from build123d import *

# Parameters (mm, degrees)
SKETCH_R        = 70
SKETCH_R_2      = 57.25
PAD_DEPTH       = 15
SKETCH001_R     = 4
SKETCH002_W     = 40
SKETCH002_H     = 40
PAD001_DEPTH    = 5
SKETCH003_R     = 2.5
POCKET_DEPTH    = 5
FILLET_R        = 18
FILLET001_R     = 11
SKETCH004_R     = 58
POCKET001_DEPTH = 15.001
SKETCH005_R     = 71
POCKET002_DEPTH = 7
SKETCH006_R     = 4
SKETCH007_R     = 105
SKETCH007_R_2   = 70
POCKET003_DEPTH = 5


with BuildPart() as part:
    # Sketch → Pad (new body)
    with BuildSketch(Plane.XY):
        Circle(SKETCH_R)
        Circle(SKETCH_R_2, mode=Mode.SUBTRACT)
    extrude(amount=PAD_DEPTH)

    # Sketch001 → Groove (revolve, cut)
    with BuildSketch(Plane.XZ):
        with Locations((63.625, 16)):
            Circle(SKETCH001_R)
    revolve(axis=Axis((0, 0, 0), (0, 0, 1)), mode=Mode.SUBTRACT)

    # Sketch002 (on Face2 of Groove) → Pad001 (join)
    with BuildSketch(Plane(origin=(0, 0, 0), x_dir=(1, 0, 0), z_dir=(0, 0, -1))):
        with Locations((82, 0)):
            Rectangle(SKETCH002_W, SKETCH002_H)
        with Locations((-82, 0)):
            Rectangle(SKETCH002_W, SKETCH002_H)
        with Locations((0, 82)):
            Rectangle(SKETCH002_W, SKETCH002_H)
        with Locations((0, -82)):
            Rectangle(SKETCH002_W, SKETCH002_H)
    extrude(amount=-PAD001_DEPTH)

    # Sketch003 (on Face13 of Pad001) → Pocket (cut)
    with BuildSketch(Plane.XY.offset(5)):
        with Locations((-86.25, 0)):
            Circle(SKETCH003_R)
        with Locations((0, -86.25)):
            Circle(SKETCH003_R)
        with Locations((86.25, 0)):
            Circle(SKETCH003_R)
        with Locations((0, 86.25)):
            Circle(SKETCH003_R)
    extrude(amount=-POCKET_DEPTH, mode=Mode.SUBTRACT)

    # Fillet
    fillet_edges = [part.edges().sort_by_distance(p)[0] for p in [
        (-20, 102, 2.5),
        (20, 102, 2.5),
        (102, 20, 2.5),
        (102, -20, 2.5),
        (20, -102, 2.5),
        (-20, -102, 2.5),
        (-102, -20, 2.5),
        (-102, 20, 2.5),
    ]]
    fillet(fillet_edges, radius=FILLET_R)

    # Fillet001
    fillet001_edges = [part.edges().sort_by_distance(p)[0] for p in [
        (67.082039, 20, 2.5),
        (20, 67.082039, 2.5),
        (-20, 67.082039, 2.5),
        (-67.082039, 20, 2.5),
        (-67.082039, -20, 2.5),
        (-20, -67.082039, 2.5),
        (20, -67.082039, 2.5),
        (67.082039, -20, 2.5),
    ]]
    fillet(fillet001_edges, radius=FILLET001_R)

    # Sketch004 (on Face41 of Fillet001) → Pocket001 (cut, through all)
    with BuildSketch(Plane.XY.offset(15)):
        Circle(SKETCH004_R)
    extrude(amount=-POCKET001_DEPTH, mode=Mode.SUBTRACT)

    # Sketch005 (on Face38 of Pocket001) → Pocket002 (cut)
    with BuildSketch(Plane.XY.offset(15)):
        Circle(SKETCH005_R)
    extrude(amount=-POCKET002_DEPTH, mode=Mode.SUBTRACT)

    # Sketch006 → Groove001 (revolve, cut)
    with BuildSketch(Plane.XZ):
        with Locations((63.625, 9)):
            Circle(SKETCH006_R)
    revolve(axis=Axis((0, 0, 0), (0, 0, 1)), mode=Mode.SUBTRACT)

    # Sketch007 (on Face37 of Groove001) → Pocket003 (cut)
    with BuildSketch(Plane.XY.offset(5)):
        Circle(SKETCH007_R)
        Circle(SKETCH007_R_2, mode=Mode.SUBTRACT)
    extrude(amount=-POCKET003_DEPTH, mode=Mode.SUBTRACT)


solid = part.part
Can you work these out from the model? Positions are in its coordinate system, mm. Coordinates: 2 decimals unless noted, no trailing zeros. Write each loop counter-clockwise with the first axis right and the second up, starting at its lowest first coordinate (ties: lowest second). Pieces come first, ordered by that corner, then holes. Notation, with made-up numbers: (12.5, 27) -> (20.5, 27) arc R27 ccw to (20.5, 55) -> close; hole circle Ø11 at (20.5, 89.25). An arc over 180 degrees is marked (long way). Write item = value, one per line.
(1) Thinking about a two-plate mould opening in X: for faces 1 (the face through (-37, 57, 8)), 2 (the face through (26.76, -51.46, 4.06)), which applies, +X half, -X half, draft (parallel to the pull), parting line (faces both ways), or undercut?
Verdict:
face_1 = draft
face_2 = undercut
(2) Imagine slicing it at B-B (z = 6.5). Please give me the cut outline in (x, y) (1 decimal).
Verdict:
outline = circle Ø140 at (0, 0); circle Ø121 at (0, 0); hole circle Ø133.5 at (0, 0); hole circle Ø116 at (0, 0)
(3) Imagine slicing it at A-A (x = 0). Please give me the cut outline in (y, z) (3 decimals), and give its area (3 significant figures).
Verdict:
outline = (-70, 0) -> (-58, 0) -> (-58, 8) -> (-59.752, 8) arc R4 cw to (-67.498, 8) -> (-70, 8) -> close; (58, 0) -> (70, 0) -> (70, 8) -> (67.498, 8) arc R4 cw to (59.752, 8) -> (58, 8) -> close
area = 158 mm^2
(4) For pin 1 (3 mm diameter, centred on x = 7, z = 6.5, fed in from -Y); pin 2 (2 mm diameter, centred on x = -27, z = 2, fed in from -Y); pin 3 (4 mm diameter, centred on y = 19, z = 5, fed in from -X), each with a flat end and sliding along its axis, tell me the tip position at first contact or that it passes through.
Verdict:
pin_1 = -69.78
pin_2 = -64.99
pin_3 = -67.9
(5) If I drill on probe 1 along X at (y, z) = (5.5, 6.75); probe 2 along Y at (x, z) = (-21.5, 7); probe 3 along X at (y, z) = (11.5, 7.25), over which ranges is the centre line in solid material (lowest first)?
Verdict:
probe_1 = -69.78 to -66.71, -60.07 to -57.74, 57.74 to 60.07, 66.71 to 69.78
probe_2 = -66.62 to -63.55, -56.19 to -53.87, 53.87 to 56.19, 63.55 to 66.62
probe_3 = -69.05 to -66.23, -58.92 to -56.85, 56.85 to 58.92, 66.23 to 69.05
